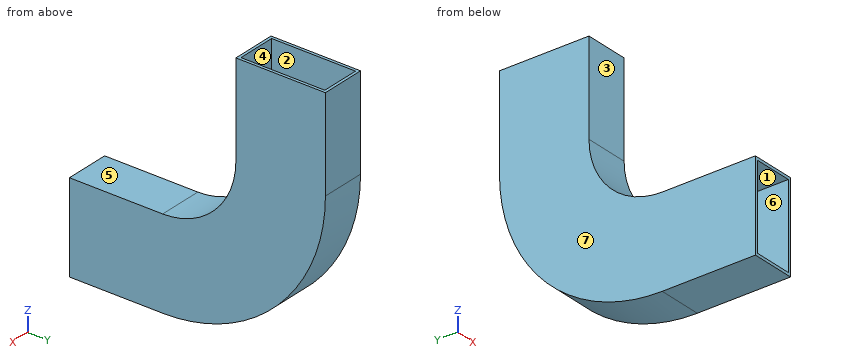
Autodesk Inventor part; units mm, degrees
ref_plane "YZ Plane" through (0, 0, 0) normal (1, 0, 0) x (0, 1, 0)
ref_plane "XZ Plane" through (0, 0, 0) normal (0, 1, 0) x (-1, 0, 0)
ref_plane "XY Plane" through (0, 0, 0) normal (0, 0, 1) x (1, 0, 0)
sketch "Sketch1" plane through (0, 0, 0) normal (0, 1, 0) x (-1, 0, 0)
  line L0 (0, 0) -> (7.899, 0)
  line L1 (7.899, 0) -> (7.899, -15.899)
  line L2 (7.899, -15.899) -> (0, -15.899)
  line L3 (0, -15.899) -> (0, 0)
  line L4 (0.5, -0.5) -> (7.399, -0.5)
  line L5 (7.399, -0.5) -> (7.399, -15.399)
  line L6 (7.399, -15.399) -> (0.5, -15.399)
  line L7 (0.5, -15.399) -> (0.5, -0.5)
  dimension "d0" = 7.899
  dimension "d1" = 15.899
  dimension "d2" = 14.899
  dimension "d3" = 6.899
  dimension "d4" = 0.5
  dimension "d5" = 0.5
sketch "Sketch3" plane through (0, 0, 0) normal (1, 0, 0) x (0, 1, 0)
  arc A0 (0, 0) -> (13, 13) centre (0, 13) ccw
  line L0 (0, 13) -> (13, 13) construction
  line L1 (0, 13) -> (0, 0) construction
  dimension "d6" = 90
  dimension "d7" = 13
sweep "Sweep1" add profiles "Sketch1" path "Sketch3"
extrude "Extrusion1" add sketch "Sketch1" against normal blind 16.55
ref_plane "Work Plane1" through (-7.899, 13, 13) normal (0, 0, 1) x (1, 0, 0)
sketch "Sketch4" plane through (-7.899, 13, 13) normal (0, 0, 1) x (1, 0, 0)
  line L0 (0, 0) -> (7.899, 0)
  line L1 (0, 0) -> (0, 15.899)
  line L2 (0, 15.899) -> (7.899, 15.899)
  line L3 (7.899, 15.899) -> (7.899, 0)
  line L4 (0.5, 15.399) -> (7.399, 15.399)
  line L5 (7.399, 15.399) -> (7.399, 0.5)
  line L6 (7.399, 0.5) -> (0.5, 0.5)
  line L7 (7.399, 0.5) -> (0.5, 0.5)
  line L8 (0.5, 0.5) -> (0.5, 15.399)
extrude "Extrusion2" add sketch "Sketch4" along normal blind 16.55
properties part number "curved waveguide"
Design review of the part built by this model. Coordinates are the model's own, in mm. Face numbers are marked on the shaded views. A direction names the side the tool comes from. Coordinates: 2 decimals unless noted, no trailing zeros. Loops run counter-clockwise (first coordinate to the right, second up) from the corner with the lowest first, then second, coordinate; pieces in that order, holes last.
Q1. For pin 1 (2 mm diameter, centred on x = -3.5, z = 18, fed in from -Y); pin 2 (3.5 mm diameter, centred on x = -3.5, y = -10, fed in from +Z); pin 3 (1 mm diameter, centred on x = -5.5, z = -7.5, fed in from -Y), all flat-tipped, find the tip position at first contact; note any pin that passes through.
Reported:
pin 1: stops at y = 13
pin 2: stops at z = 0
pin 3: stops at y = 19.12
Q2. Tool access review of the marked faces 1, 2 and 3: name each direction out of +Z, -Z, +X, -X, +Y, -Y from which nothing blocks a thin tool from reaching the whole face with its end or side.
Reported:
face 1: -Y
face 2: none
face 3: +Z, +X, -X, -Y
Q3. The part is to be moulded in two halves that separate along X. For the marked faces 4, 5, 6 and 7, say which applies: +X half, -X half, draft (parallel to the pull), parting line (faces both ways), or undercut.
Reported:
face 4: undercut
face 5: draft
face 6: undercut
face 7: -X half
Q4. We need section D-D on z = -3.5. State the section outline as (x, y) points.
Reported:
outline: (-7.9, -16.55) - (-7.4, -16.55) - (-7.4, 23.11) - (-0.5, 23.11) - (-0.5, -16.55) - (0, -16.55) - (0, 23.73) - (-7.9, 23.73) - close
Q5. We need section A-A on y = -5. State the section outline as (x, z) points, and give its area (3 significant figures).
Reported:
outline: (-7.9, -15.9) - (0, -15.9) - (0, 0) - (-7.9, 0) - close; hole (-7.4, -15.4) - (-0.5, -15.4) - (-0.5, -0.5) - (-7.4, -0.5) - close
area: 22.8 mm2
Q6. We need section B-B on x = -3.5. State the section outline as (y, z) points.
Reported:
outline: (-16.55, -15.9) - (0, -15.9) arc R28.9 ccw to (28.9, 13) - (28.9, 29.55) - (28.4, 29.55) - (28.4, 13) arc R28.4 cw to (0, -15.4) - (-16.55, -15.4) - close; (-16.55, -0.5) - (0, -0.5) arc R13.5 ccw to (13.5, 13) - (13.5, 29.55) - (13, 29.55) - (13, 13) arc R13 cw to (0, 0) - (-16.55, 0) - close
Q7. To check wall thickness, follow line 1 (X direction, y = -10, z = -9); line 2 (Z direction, x = -4, y = -9); line 3 (Y direction, x = -3.5, z = 25.5). State the ranges of each line that lie inside material, in increasing order.
Reported:
line 1: x = -7.9 to -7.4, -0.5 to 0
line 2: z = -15.9 to -15.4, -0.5 to 0
line 3: y = 13 to 13.5, 28.4 to 28.9
Q8. We need section C-C on z = 20.5. State the section outline as (x, y) points, and give its area (3 significant figures).
Reported:
outline: (-7.9, 13) - (0, 13) - (0, 28.9) - (-7.9, 28.9) - close; hole (-7.4, 13.5) - (-0.5, 13.5) - (-0.5, 28.4) - (-7.4, 28.4) - close
area: 22.8 mm2
